Build history of the part. All positions in model axes, mm. Give positions to 0.01 mm unless a question says otherwise; leave off trailing zeros. Order: outer loops, then holes, each group sorted by start corner. A loop starts at its lowest first (then second) coordinate and runs counter-clockwise, first axis right, second up. Notation, with made-up numbers: (20.5, 68.25) - (42.5, 68.25) arc R13 ccw to (42.5, 78.25) - close; hole circle Ø6 at (23, 45.25). An arc over 180 degrees is marked (long way). Use a Markdown table: item, result. Add a question column.
(1) Flat gauge pins, fed straight in: pin 1 (3 mm diameter, centred on x = 38.5, y = 0.5, fed in from +Z); pin 2 (4 mm diameter, centred on y = -0.5, z = -1.5, fed in from -X); pin 3 (2 mm diameter, centred on x = 14.5, y = -1.5, fed in from -Z); pin 4 (2 mm diameter, centred on x = 15, z = 1.5, fed in from +Y). Where does each tip first touch, or does it go through?
(2) Wall check: line 1 (X direction, y = 1, z = 3.5); line 2 (Z direction, x = 16.5, y = 0.25); line 3 (Y direction, x = 13.5, z = 0). Give the ranges that are in metal, low to high.
(3) Mould opens along X. For faces 1 (the face through (29.58, -2.44, 0.54)), 2 (the face through (60, 3, 0)), 3 (the face through (-1.7, 0, 0)), 4 (the face through (61.7, 0, 0)) say: +X half, -X half, draft (parallel to the pull), parting line (faces both ways), or undercut.
(4) Slice it at A-A (x = 8). Write the cut outline in (y, z), then the cut area to 3 significant figures.
from build123d import *

# Parameters (mm, degrees)
SKETCH_1_R      = 2.5
EXTRUDE_1_DEPTH = 60
SKETCH_2_R      = 3.95
EXTRUDE_2_DEPTH = 1.7
EXTRUDE_START   = 1.7
SKETCH_3_R      = 3.95
EXTRUDE_3_DEPTH = 1.7
FILLET_1_R      = 3.9


with BuildPart() as part:
    # Эскиз1 → Бобышка-Вытянуть1 (new body)
    with BuildSketch(Plane(origin=(0, 0, 0), x_dir=(0, 0, -1), z_dir=(1, 0, 0))):
        Circle(SKETCH_1_R)
    extrude(amount=EXTRUDE_1_DEPTH)

    # Эскиз2 → Бобышка-Вытянуть2 (add)
    with BuildSketch(Plane.ZY):
        Circle(SKETCH_2_R)
    extrude(amount=EXTRUDE_2_DEPTH)

    # Эскиз3 → Бобышка-Вытянуть3 (add)
    with BuildSketch(Plane(origin=(60, 0, 0), x_dir=(0, 0, -1), z_dir=(1, 0, 0)).offset(EXTRUDE_START)):
        with Locations(Location((0, 0, 0), (0, 0, 180))):
            Circle(SKETCH_3_R)
    extrude(amount=-EXTRUDE_3_DEPTH)

    # Скругление1
    # the kernel refuses this fillet: 3.9 mm, written as the material it takes off along each edge
    with BuildSketch(Plane(origin=(61.7, 0, 0), x_dir=(0, 0, 1), z_dir=(0, 1, 0))) as fillet_1_piece_1:
        with BuildLine():
            CenterArc((0.729751562, -3.9), FILLET_1_R, 34.339994944, 55.660005056)
            Line((0.729751562, 0), (0.729751562, 0.078))
            Line((0.729751562, 0.078), (3.95, 0.078))
            Line((3.95, 0.078), (4.028, 0))
            ThreePointArc((4.028, 0), (4.028, -0.85), (4.014404969, -1.656))
            Line((4.014404969, -1.656), (3.95, -1.7))
        make_face()
    revolve(axis=Axis((61.7, 0, 0), (1, 0, 0)), mode=Mode.SUBTRACT)
    with BuildSketch(Plane(origin=(-1.7, 0, 0), x_dir=(0, 0, 1), z_dir=(0, -1, 0))) as fillet_1_piece_2:
        with BuildLine():
            CenterArc((0.729751562, -3.9), FILLET_1_R, 34.339994944, 55.660005056)
            Line((0.729751562, 0), (0.729751562, 0.078))
            Line((0.729751562, 0.078), (3.95, 0.078))
            Line((3.95, 0.078), (4.028, 0))
            ThreePointArc((4.028, 0), (4.028, -0.85), (4.014404969, -1.656))
            Line((4.014404969, -1.656), (3.95, -1.7))
        make_face()
    revolve(axis=Axis((-1.7, 0, 0), (-1, 0, 0)), mode=Mode.SUBTRACT)


solid = part.part
Solution:
| question | item | result |
|---|---|---|
| 1 | pin 1 | z = 2.5 |
| 1 | pin 2 | x = -1.7 |
| 1 | pin 3 | z = -2.45 |
| 1 | pin 4 | y = 2.45 |
| 2 | line 1 | -0.4 to 0, 60 to 60.4 |
| 2 | line 2 | -2.49 to 2.49 |
| 2 | line 3 | -2.5 to 2.5 |
| 3 | face 1 | undercut |
| 3 | face 2 | undercut |
| 3 | face 3 | -X half |
| 3 | face 4 | +X half |
| 4 | outline | circle Ø5 at (0, 0) |
| 4 | area | 19.6 mm2 |
